For this review, take the finished solid that the model builds, in its own axes (mm). A direction names the side the tool comes from. Give positions to 0.01 mm unless a question says otherwise; leave off trailing zeros. Write each loop counter-clockwise with the first axis right and the second up, starting at its lowest first coordinate (ties: lowest second). Pieces come first, ordered by that corner, then holes.
Q1. We need section C-C (z = -119). Write out the cut boundary in (x, y).
Q2. Mouldability with a two-part tool opening along Y and no side actions: class faces 5 (the flat face through (-29, -22.5, -120)), 6 (the cylindrical face through (17.13, -58.52, 20.87)), 7 (the cylindrical face through (-39.4, -2.17, -182.75)) as released by +Y, released by -Y, zero draft, split by the parting line, or undercut.
Q3. We need section D-D (y = -31.5). Write out the cut boundary in (x, z).
Q4. Insertion check: P1, Ø22.5, axis at y = 3, z = -112.5, coming from the +X side; P2, Ø15.5, axis at x = -34, z = -100.5, coming from the -Y side; P3, Ø2, axis at x = -12, y = -9.5, coming from the +Z side; P4, Ø22, axis at x = -30, y = -1, coming from the -Z side. Each pin has a flat end and moves straight along its axis. Give the tip position at first contact, or say it passes through.
Q5. We need section A-A (z = 0). Write out the cut boundary in (x, y).
Q6. We need section B-B (y = 0). Write out the cut boundary in (x, z), then the cut area to 3 significant figures.
Q7. For line 1 (X direction, y = 0, z = -184); line 2 (Y direction, x = -46, z = -175.5); line 3 (Y direction, x = -18, z = -8), list the stretches that pass through material, from the lowest coordinate up.
Q8. Machinability: for faces 1 (the flat face through (-29, 0, -177.676)), 2 (the flat face through (-4.138, 0, -118)), 3 (the flat face through (-55.138, 0, -120)), 4 (the flat face through (-14, 57, -17)), which of the approach directions +Z, -Z, +X, -X, +Y, -Y give a long, thin tool a straight path to every point of the face, cutting with its end or side? Answer none if there is none.
Autodesk Inventor part; units mm, degrees
ref_plane "YZ Plane" through (0, 0, 0) normal (1, 0, 0) x (0, 1, 0)
ref_plane "XZ Plane" through (0, 0, 0) normal (0, 1, 0) x (-1, 0, 0)
ref_plane "XY Plane" through (0, 0, 0) normal (0, 0, 1) x (1, 0, 0)
sketch "Sketch1" plane through (0, 0, 0) normal (1, 0, 0) x (0, 1, 0)
  circle A0 centre (0, 0) radius 10
  line L0 (0, 0) -> (-50.6762, -56.6385) construction
  line L1 (-50.6762, -56.6385) -> (-50.6762, -2.6385)
  line L2 (-50.6762, -56.6385) -> (-23.6762, -56.6385)
  arc A1 (17.7921, -20.3086) -> (-15.5352, 22.083) centre (0, 0) ccw
  line L3 (-50.6762, -2.6385) -> (-15.5352, 22.083)
  line L4 (-23.6762, -56.6385) -> (17.7921, -20.3086)
  dimension "d0" = 20
  dimension "d2" = 41.82
  dimension "d5" = 76
  dimension "d6" = 27
  dimension "d7" = 54
  dimension "d8" = 54
extrude "Extrusion1" add sketch "Sketch1" along normal mid plane 120
sketch "Sketch2" plane through (0, 0, 0) normal (1, 0, 0) x (0, 1, 0)
  circle A0 centre (0, 0) radius 10
  line L0 (-50.6762, -2.6385) -> (-50.6762, -56.6385)
  line L1 (-50.6762, -56.6385) -> (-23.6762, -56.6385)
  line L2 (-23.6762, -56.6385) -> (17.7921, -20.3086)
  arc A1 (17.7921, -20.3086) -> (-15.5352, 22.083) centre (0, 0) ccw
  line L3 (-15.5352, 22.083) -> (-50.6762, -2.6385)
  line L4 (-44.6762, -56.6385) -> (-44.6762, 1.5825)
  line L5 (-44.6762, 1.5825) -> (-15.5352, 22.083)
  line L6 (-44.6762, -56.6385) -> (-23.6762, -56.6385)
  dimension "d11" = 6
extrude "Extrusion2" cut sketch "Sketch2" along normal mid plane 114 contours L3 A1 L2 L1 L4
sketch "Sketch3" plane through (0, 0, 0) normal (1, 0, 0) x (0, 1, 0)
  line L0 (-50.6762, -29.6385) -> (-80.5956, -29.6385) construction
  line L1 (-50.6762, -2.6385) -> (-50.6762, -56.6385)
  line L2 (-50.6762, -4.1385) -> (-187.6762, -4.1385)
  line L3 (-187.6762, -4.1385) -> (-187.6762, -55.1385)
  line L4 (-187.6762, -55.1385) -> (-50.6762, -55.1385)
  line L5 (-50.6762, -55.1385) -> (-50.6762, -4.1385)
  line L6 (-50.6762, -29.6385) -> (-187.6762, -29.6385) construction
  point P0 (0, 0)
  dimension "d14" = 51
  dimension "d16" = 137
extrude "Extrusion3" add sketch "Sketch3" along normal mid plane 45
sketch "Sketch5" plane through (-22.5, -187.6762, -55.1385) normal (0, -1, 0) x (1, 0, 0)
  line L0 (0, 51) -> (45, 0) construction
  circle A0 centre (22.5, 25.5) radius 10
  point P0 (22.5, 55.1385)
  dimension "d19" = 20
extrude "Extrusion4" cut sketch "Sketch5" against normal blind 10
move or copy body "Move Body6" bodies to move or copy 1 copy no rotation origin (0, 0, 0) rotation axis (1, 0, 0) rotation angle 90
move or copy body "Move Body7" bodies to move or copy 1 copy no rotation origin (0, 0, 0) rotation axis (0, 0, 1) rotation angle 90
properties part number "Elbow_Pitch"
Computed:
1. outline: (-55.14, -22.5) - (-4.14, -22.5) - (-4.14, 22.5) - (-55.14, 22.5) - close
2. face 5: released by -Y
2. face 6: zero draft
2. face 7: undercut
3. outline: (-56.64, -50.68) - (-2.64, -50.68) - (1.58, -44.68) - (-56.64, -44.68) - close
4. P1: stops at x = -4.14
4. P2: stops at y = -22.5
4. P3: stops at z = -44.68
4. P4: stops at z = -187.68
5. outline: (-35.9, -60) - (-10, -60) - (-10, -57) - (-35.9, -57) - close; (-35.9, 57) - (-10, 57) - (-10, 60) - (-35.9, 60) - close; (10, -60) - (27, -60) - (27, -57) - (10, -57) - close; (10, 57) - (27, 57) - (27, 60) - (10, 60) - close
6. outline: (-56.64, -50.68) - (-55.14, -50.68) - (-55.14, -187.68) - (-39.64, -187.68) - (-39.64, -177.68) - (-19.64, -177.68) - (-19.64, -187.68) - (-4.14, -187.68) - (-4.14, -50.68) - (-2.64, -50.68) - (1.58, -44.68) - (-56.64, -44.68) - close
6. area: 7,120 mm2
7. line 1: x = -55.14 to -39.64, -19.64 to -4.14
7. line 2: y = -22.5 to 22.5
7. line 3: y = -60 to -57, 57 to 60
8. face 1: -Z
8. face 2: -Z, +X, +Y, -Y
8. face 3: -Z, -X, +Y, -Y
8. face 4: +Z, +X, -X
